```python
from build123d import *

# Parameters (mm, degrees)
SKIZZE1_W                             = 15
SKIZZE1_H                             = 30
AUFSATZ_LINEAR_AUSTRAGEN1_DEPTH       = 10
FORMSENKUNG_F_R_M4_SFHCS1_D           = 4.5
FORMSENKUNG_F_R_M4_SFHCS1_CSINK_D     = 8.96
FORMSENKUNG_F_R_M4_SFHCS1_CSINK_ANGLE = 90
SKIZZE4_R                             = 3.1
SCHNITT_LINEAR_AUSTRAGEN1_DEPTH       = 4
SKIZZE7_R                             = 4
SCHNITT_LINEAR_AUSTRAGEN2_DEPTH       = 6
M3X0_5_GEWINDEBOHRUNG1_D              = 2.5
M3X0_5_GEWINDEBOHRUNG1_CSINK_D        = 3.05
M3X0_5_GEWINDEBOHRUNG1_CSINK_ANGLE    = 90


with BuildPart() as part:
    # Skizze1 → Aufsatz-Linear austragen1 (new body)
    with BuildSketch(Plane.XY):
        with Locations((7.5, 15)):
            Rectangle(SKIZZE1_W, SKIZZE1_H)
    extrude(amount=AUFSATZ_LINEAR_AUSTRAGEN1_DEPTH)

    # Formsenkung für M4 SFHCS1 (through all)
    with Locations(Plane.XY.offset(10)):
        with Locations((7.5, 25), (7.5, 5)):
            CounterSinkHole(FORMSENKUNG_F_R_M4_SFHCS1_D / 2, FORMSENKUNG_F_R_M4_SFHCS1_CSINK_D / 2, counter_sink_angle=FORMSENKUNG_F_R_M4_SFHCS1_CSINK_ANGLE)

    # Skizze4 → Schnitt-Linear austragen1 (cut)
    with BuildSketch(Plane(origin=(0, 0, 0), x_dir=(-1, 0, 0), z_dir=(0, 0, -1))):
        with Locations((-7.5, 25)):
            Circle(SKIZZE4_R)
        with Locations((-7.5, 5)):
            Circle(SKIZZE4_R)
    extrude(amount=-SCHNITT_LINEAR_AUSTRAGEN1_DEPTH, mode=Mode.SUBTRACT)

    # Skizze7 → Schnitt-Linear austragen2 (cut)
    with BuildSketch(Plane.XY.offset(10)):
        with Locations((7.5, 15)):
            Circle(SKIZZE7_R)
    extrude(amount=-SCHNITT_LINEAR_AUSTRAGEN2_DEPTH, mode=Mode.SUBTRACT)

    # M3x0.5 Gewindebohrung1 (through all)
    with Locations(Plane(origin=(15, 0, 0), x_dir=(0, 0, -1), z_dir=(1, 0, 0))):
        with Locations((-7, 15)):
            CounterSinkHole(M3X0_5_GEWINDEBOHRUNG1_D / 2, M3X0_5_GEWINDEBOHRUNG1_CSINK_D / 2, counter_sink_angle=M3X0_5_GEWINDEBOHRUNG1_CSINK_ANGLE)


solid = part.part
```
Input: part model. Units: mm. Frame: model coordinates. A direction names the side the tool comes from. Coordinates: 2 decimals unless noted, no trailing zeros. Loops run counter-clockwise (first coordinate to the right, second up) from the corner with the lowest first, then second, coordinate; pieces in that order, holes last. Notation, with made-up numbers: M 58.25,53 L 108.25,53 A19 cw 108.25,79 Z; hole C 13.5,62 d6. An arc over 180 degrees is marked long. Use a Markdown table: item, result. Add a question column.
1) Pin query (flat end, axial travel): P1, Ø3, axis at y = 15, z = 7, coming from the -X side; P2, Ø2.5, axis at x = 7, y = 16.5, coming from the +Z side; P3, Ø6, axis at x = 7.5, y = 25, coming from the +Z side. Return the tip coordinate at first contact, or that it passes through.
2) Section D-D, the plane x = 14. Return the cut outline in (y, z).
3) Section C-C, the plane x = 7.5. Return the cut outline in (y, z).
4) Draft query along X for faces 4 (the flat face through (0, 15, 5)), 5 (the flat face through (5, 26, 4)), 6 (the flat face through (7, 30, 5)). Return one class per face: +X half, -X half, draft (parallel to the pull), parting line (faces both ways), or undercut.
5) Line query: L1, parallel to Y at x = 7.5, z = 6; L2, parallel to Y at x = 7.5, z = 2.95; L3, parallel to Z at x = 1.9, y = 15. Output: solid intervals per line, ascending. Write a range as from..to.
6) Set-up query: faces 1 (the flat face through (7, 0, 5)), 2 (the flat face through (5, 6, 4)), 3 (the flat face through (7, 15, 4)). Return all of +Z, -Z, +X, -X, +Y, -Y with unobstructed straight access to the full face (end or side cutting, diameter ignored); none if empty.
7) Section A-A, the plane z = 7. Return the cut outline in (x, y) (3 decimals).
8) Section B-B, the plane y = 5. Return the cut outline in (x, z).
Answer below:
| question | item | result |
|---|---|---|
| 1 | P1 | x = 0 |
| 1 | P2 | z = 4 |
| 1 | P3 | z = 8.52 |
| 2 | outline | M 0,0 L 30,0 L 30,10 L 0,10 Z; hole C 15,7 d2.5 |
| 3 | outline | M 0,0 L 1.9,0 L 1.9,4 L 2.75,4 L 2.75,7.77 L 0.52,10 L 0,10 Z; M 7.25,4 L 8.1,4 L 8.1,0 L 21.9,0 L 21.9,4 L 22.75,4 L 22.75,7.77 L 20.52,10 L 19,10 L 19,4 L 11,4 L 11,10 L 9.48,10 L 7.25,7.77 Z; M 27.25,4 L 28.1,4 L 28.1,0 L 30,0 L 30,10 L 29.48,10 L 27.25,7.77 Z |
| 4 | face 4 | -X half |
| 4 | face 5 | undercut |
| 4 | face 6 | draft |
| 5 | L1 | 0..2.75, 7.25..11, 19..22.75, 27.25..30 |
| 5 | L2 | 0..1.9, 8.1..21.9, 28.1..30 |
| 5 | L3 | 0..5.75, 8.25..10 |
| 6 | face 1 | +Z, -Z, +X, -X, -Y |
| 6 | face 2 | -Z |
| 6 | face 3 | +Z |
| 7 | outline | M 0,0 L 15,0 L 15,13.475 L 14.725,13.75 L 11.3,13.75 A4 cw 3.7,13.75 L 0,13.75 Z; M 0,16.25 L 3.7,16.25 A4 cw 11.3,16.25 L 14.725,16.25 L 15,16.525 L 15,30 L 0,30 Z; hole C 7.5,5 d4.5; hole C 7.5,25 d4.5 |
| 8 | outline | M 0,0 L 4.4,0 L 4.4,4 L 5.25,4 L 5.25,7.77 L 3.02,10 L 0,10 Z; M 9.75,4 L 10.6,4 L 10.6,0 L 15,0 L 15,10 L 11.98,10 L 9.75,7.77 Z |
